Geometry check sheet. Reference: drawing and pictorial views, mm from the part's lowest x, y, z. Round coordinates to 2 decimals unless told otherwise and drop trailing zeros. Write each loop counter-clockwise with the first axis right and the second up, starting at its lowest first coordinate (ties: lowest second). Pieces come first, ordered by that corner, then holes. Notation, with made-up numbers: M -25.75,1 L -5.75,1 A15 cw -5.75,7 Z; hole C 77.25,6 d3. An arc over 180 degrees is marked long. One line per question, with ' | ' between items.
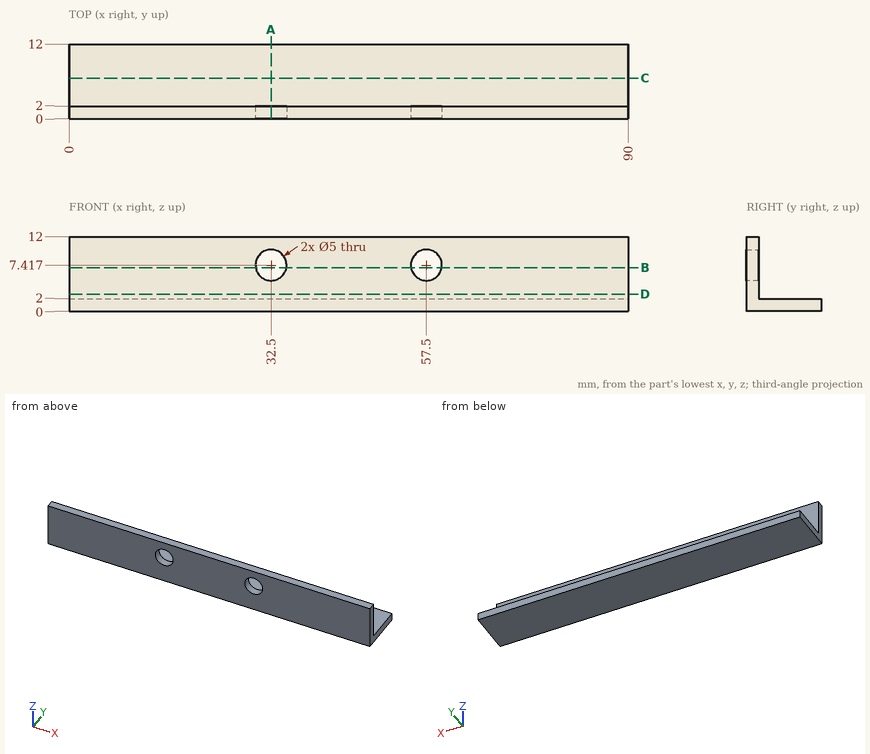
1. Section check C-C, the plane y = 6.5. Record the cut outline in (x, z), then the cut area to 3 significant figures.
Results:
outline: M 0,0 L 90,0 L 90,2 L 0,2 Z | area: 180 mm2
2. Thickness scan on line 1 (Z direction, x = 32.5, y = 0.45); line 2 (Z direction, x = 46, y = 10.75). Record the ranges inside material, lowest first.
Results:
line 1: z = 0 to 4.92, 9.92 to 12 | line 2: z = 0 to 2
3. Go/stop test with flat-tipped pins: P1, Ø1.5, axis at x = 39.5, z = 6, coming from the -Y side; P2, Ø6, axis at x = 32.5, z = 7.42, coming from the +Y side; P3, Ø3, axis at x = 61.5, y = 7.5, coming from the +Z side. Record where each tip stops, or that it passes through.
Results:
P1: stops at y = 0 | P2: stops at y = 2 | P3: stops at z = 2
4. Section check B-B, the plane z = 7. Record the cut outline in (x, y) (1 decimal), then the cut area to 3 significant figures.
Results:
outline: M 0,0 L 30,0 L 30,2 L 0,2 Z; M 35,0 L 55,0 L 55,2 L 35,2 Z; M 60,0 L 90,0 L 90,2 L 60,2 Z | area: 160 mm2
5. Section check A-A, the plane x = 32.5. Record the cut outline in (y, z), then the cut area to 3 significant figures.
Results:
outline: M 0,0 L 12,0 L 12,2 L 2,2 L 2,4.92 L 0,4.92 Z; M 0,9.92 L 2,9.92 L 2,12 L 0,12 Z | area: 34.0 mm2
